```python
from build123d import *

# Parameters (mm, degrees)
F1_DEPTH        = 17.5
F2_DEPTH        = 12
F3_DEPTH        = 3.5
F4_R            = 10
F7_R            = 10
F11_D           = 9
F13_D           = 9
F20_D           = 5.5
F20_DEPTH       = 3.5
F20_CSINK_D     = 8
F20_CSINK_ANGLE = 82
F20_TIP         = 1.6523667023
F22_D           = 5.5
F22_DEPTH       = 3.5
F22_CSINK_D     = 8
F22_CSINK_ANGLE = 82
F22_TIP         = 1.6523667023
F24_DEPTH       = 2.5


with BuildPart() as f1:
    # F0 (on Front) → F1 (new body, symmetric)
    with BuildSketch(Plane.XZ):
        Polygon((52, -6), (52, 6), (23.1059112473, 6), (16.606986017, 6), (9.0432994782, 6), (7.106986017, 6), (-9.5, 6), (-29.3893709637, 6), (-52, 6), (-52, -6), align=None)
    extrude(amount=F1_DEPTH, both=True)

    # F0 (on Front) → F2 (join, symmetric)
    with BuildSketch(Plane.XZ):
        with BuildLine():
            ThreePointArc((-24.5597418322, 9.7059047745), (-26.3455638186, 7.0332332985), (-29.3893709637, 6))
            Line((-29.3893709637, 6), (-9.5, 6))
            Line((-9.5, 6), (-9.5, 26))
            Line((-9.5, 26), (-15, 26))
            ThreePointArc((-15, 26), (-17.9660849945, 25.5499916129), (-20.665217364, 24.2404679611))
            Line((-20.665217364, 24.2404679611), (-24.5597418322, 9.7059047745))
        make_face()
        with BuildLine():
            ThreePointArc((-11, 16), (-17.8284271247, 13.1715728753), (-15, 20))
            ThreePointArc((-15, 20), (-12.1715728753, 18.8284271247), (-11, 16))
        make_face(mode=Mode.SUBTRACT)
        with BuildLine():
            Line((-9.5, 6), (7.106986017, 6))
            ThreePointArc((7.106986017, 6), (4.7982429508, 6.5649458341), (3.0112257955, 8.1321178182))
            Line((3.0112257955, 8.1321178182), (-9.5, 26))
            Line((-9.5, 26), (-9.5, 6))
        make_face()
        with BuildLine():
            Line((9.0432994782, 6), (16.606986017, 6))
            ThreePointArc((16.606986017, 6), (14.2982429508, 6.5649458341), (12.5112257955, 8.1321178182))
            Line((12.5112257955, 8.1321178182), (0, 26))
            Line((0, 26), (-9.5, 26))
            Line((-9.5, 26), (3.0112257955, 8.1321178182))
            ThreePointArc((3.0112257955, 8.1321178182), (4.7982429508, 6.5649458341), (7.106986017, 6))
            Line((7.106986017, 6), (9.0432994782, 6))
        make_face()
    extrude(amount=F2_DEPTH, both=True)

    # F0 (on Front) → F3 (join, symmetric)
    with BuildSketch(Plane.XZ):
        with BuildLine():
            Line((16.606986017, 6), (23.1059112473, 6))
            ThreePointArc((23.1059112473, 6), (20.7971681811, 6.5649458341), (19.0101510258, 8.1321178182))
            Line((19.0101510258, 8.1321178182), (-2.4481396714, 38.7777329056))
            ThreePointArc((-2.4481396714, 38.7777329056), (-10.4179907667, 42.9471562808), (-17.2274066103, 37.0705523608))
            Line((-17.2274066103, 37.0705523608), (-20.665217364, 24.2404679611))
            ThreePointArc((-20.665217364, 24.2404679611), (-17.9660849945, 25.5499916129), (-15, 26))
            Line((-15, 26), (-9.5, 26))
            Line((-9.5, 26), (0, 26))
            Line((0, 26), (12.5112257955, 8.1321178182))
            ThreePointArc((12.5112257955, 8.1321178182), (14.2982429508, 6.5649458341), (16.606986017, 6))
        make_face()
        with BuildLine():
            ThreePointArc((-6.75, 35), (-7.5554563517, 33.0554563517), (-9.5, 32.25))
            ThreePointArc((-9.5, 32.25), (-11.4445436483, 36.9445436483), (-6.75, 35))
        make_face(mode=Mode.SUBTRACT)
    extrude(amount=F3_DEPTH, both=True)

    # F8: sweep along a path in F5
    with BuildLine(Plane.XZ.offset(12)) as f8_path:
        Line((0, 26), (14.0041507642, 6))
    # F4 (on face) → F8 (sweep, cut)
    with BuildSketch(Plane.XY.offset(26)):
        with Locations((0, -13.5)):
            Circle(F4_R)
    sweep(path=f8_path.line, mode=Mode.SUBTRACT)

    # F9: sweep along a path in F6
    with BuildLine(Plane(origin=(0, 12, 0), x_dir=(-1, 0, 0), z_dir=(0, 1, 0))) as f9_path:
        Line((0, 26), (-14.0041507642, 6))
    # F7 (on face) → F9 (sweep, cut)
    with BuildSketch(Plane.XY.offset(26)):
        with Locations((0, 13.5)):
            Circle(F7_R)
    sweep(path=f9_path.line, mode=Mode.SUBTRACT)

    # F11 (through all)
    with Locations(Plane.XY.offset(6)):
        with Locations((40, 0)):
            Hole(F11_D / 2)

    # F13 (through all)
    with Locations(Plane.XY.offset(6)):
        with Locations((-40, 0)):
            Hole(F13_D / 2)

    # F15: sweep along a path in F15_path
    with BuildLine(Plane(origin=(-52, -17.5, -6), x_dir=(0, 0, -1), z_dir=(0, 1, 0))) as f15_path:
        Line((0, 0), (-12, 0))
    # F14 (on face) → F15 (sweep, cut)
    with BuildSketch(Plane.XY.offset(6)):
        with BuildLine():
            Line((-45.3612986682, 10.6920782903), (-32, 17.5))
            Line((-32, 17.5), (-52, 17.5))
            Line((-52, 17.5), (-52, -17.5))
            Line((-52, -17.5), (-32, -17.5))
            Line((-32, -17.5), (-45.3612986682, -10.6920782903))
            ThreePointArc((-45.3612986682, -10.6920782903), (-51.9134126713, 0), (-45.3612986682, 10.6920782903))
        make_face()
    sweep(path=f15_path.line, mode=Mode.SUBTRACT)

    # F16: sweep along a path in F0
    with BuildLine(Plane.XZ) as f16_path:
        Line((-52, 6), (-52, -6))
    # F12 (on face) → F16 (sweep, cut)
    with BuildSketch(Plane.XY.offset(6)):
        with BuildLine():
            ThreePointArc((-40, -4.5), (-44.5, 0), (-40, 4.5))
            Line((-40, 4.5), (-52, 4.5))
            Line((-52, 4.5), (-52, -4.5))
            Line((-52, -4.5), (-40, -4.5))
        make_face()
    sweep(path=f16_path.line, mode=Mode.SUBTRACT)

    # F17: sweep along a path in F17_path
    with BuildLine(Plane(origin=(52, 17.5, 6), x_dir=(0, 0, 1), z_dir=(0, -1, 0))) as f17_path:
        Line((0, 0), (-12, 0))
    # F12 (on face) → F17 (sweep, cut)
    with BuildSketch(Plane.XY.offset(6)):
        with BuildLine():
            Line((45.3612986682, -10.6920782903), (32, -17.5))
            Line((32, -17.5), (52, -17.5))
            Line((52, -17.5), (52, -4.4991668823))
            Line((52, -4.4991668823), (51.0380473784, -4.4991668823))
            ThreePointArc((51.0380473784, -4.4991668823), (48.7593240742, -8.1086282103), (45.3612986682, -10.6920782903))
        make_face()
    sweep(path=f17_path.line, mode=Mode.SUBTRACT)

    # F18: sweep along a path in F18_path
    with BuildLine(Plane(origin=(52, 17.5, 6), x_dir=(0, 0, 1), z_dir=(0, -1, 0))) as f18_path:
        Line((0, 0), (-12, 0))
    # F12 (on face) → F18 (sweep, cut)
    with BuildSketch(Plane.XY.offset(6)):
        with BuildLine():
            ThreePointArc((51.0380473784, -4.4991668823), (51.9134126713, 0), (51.0380473784, 4.4991668823))
            Line((51.0380473784, 4.4991668823), (40.0865873287, 4.4991668823))
            ThreePointArc((40.0865873287, 4.4991668823), (43.2124478968, 3.1512185755), (44.5, 0))
            ThreePointArc((44.5, 0), (43.2124478968, -3.1512185755), (40.0865873287, -4.4991668823))
            Line((40.0865873287, -4.4991668823), (51.0380473784, -4.4991668823))
        make_face()
        with BuildLine():
            Line((52, 4.4991668823), (51.0380473784, 4.4991668823))
            ThreePointArc((51.0380473784, 4.4991668823), (51.9134126713, 0), (51.0380473784, -4.4991668823))
            Line((51.0380473784, -4.4991668823), (52, -4.4991668823))
            Line((52, -4.4991668823), (52, 4.4991668823))
        make_face()
        with BuildLine():
            Line((52, 17.5), (32, 17.5))
            Line((32, 17.5), (45.3612986682, 10.6920782903))
            ThreePointArc((45.3612986682, 10.6920782903), (48.7593240742, 8.1086282103), (51.0380473784, 4.4991668823))
            Line((51.0380473784, 4.4991668823), (52, 4.4991668823))
            Line((52, 4.4991668823), (52, 17.5))
        make_face()
    sweep(path=f18_path.line, mode=Mode.SUBTRACT)

    # F20
    with Locations(Plane.XZ.offset(3.5)):
        with Locations((-9.5, 35)):
            CounterSinkHole(F20_D / 2, F20_CSINK_D / 2, depth=F20_DEPTH, counter_sink_angle=F20_CSINK_ANGLE)
            with Locations((0, 0, -(F20_DEPTH + F20_TIP / 2))):  # 118° drill point
                Cone(0, F20_D / 2, F20_TIP, mode=Mode.SUBTRACT)

    # F22
    with Locations(Plane(origin=(0, 3.5, 0), x_dir=(-1, 0, 0), z_dir=(0, 1, 0))):
        with Locations((9.5, 35)):
            CounterSinkHole(F22_D / 2, F22_CSINK_D / 2, depth=F22_DEPTH, counter_sink_angle=F22_CSINK_ANGLE)
            with Locations((0, 0, -(F22_DEPTH + F22_TIP / 2))):  # 118° drill point
                Cone(0, F22_D / 2, F22_TIP, mode=Mode.SUBTRACT)

    # F23 (on Front) → F24 (cut, symmetric)
    with BuildSketch(Plane.XZ):
        Polygon((-13.4935649536, 32.709419195), (-9.5146586694, 30.3951730687), (-5.5210095913, 32.6838839269), (-5.5062667973, 37.2868409115), (-9.4851730816, 39.6010870379), (-13.4788221597, 37.3123761796), align=None)
    extrude(amount=F24_DEPTH, both=True, mode=Mode.SUBTRACT)


solid = f1.part
```
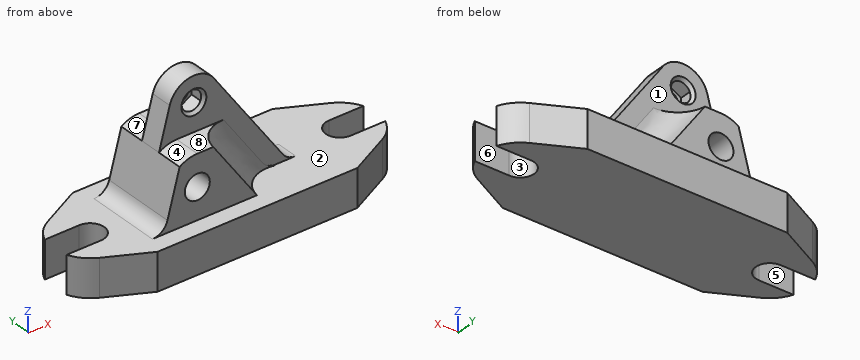
Check sheet for the modelled part. Datum: model origin and axes. Units: mm. Face numbers are marked on the shaded views. A direction names the side the tool comes from. Give positions to 0.01 mm unless a question says otherwise; leave off trailing zeros. Write each loop counter-clockwise with the first axis right and the second up, starting at its lowest first coordinate (ties: lowest second). Pieces come first, ordered by that corner, then holes.
Item 1: Cross-section at B-B (x = -42). Enter the section's corners in (y, z), and give its area (3 significant figures).
Item 2: Access from +Z, -Z, +X, -X, +Y, -Y to the whole of each face (thin tool, end or side, straight path). Record for the marked faces 4, 5, 6, 7 and 8.
Item 3: Cross-section at D-D (x = 20.5). Enter the section's corners in (y, z).
Item 4: Gauge pin test, flat ends, axial feed: pin 1 (5.5 mm diameter, centred on x = 48.5, z = -1, fed in from -Y); pin 2 (4 mm diameter, centred on x = -8.5, z = 33.5, fed in from +Y); pin 3 (3 mm diameter, centred on y = 8, z = 3.5, fed in from -X); pin 4 (16 mm diameter, centred on x = -18.5, z = 12, fed in from +Y). Record the tip position at first contact, or that the pin passes through.
Item 5: Scan lines: L1, parallel to Z at x = -15, y = -4; L2, parallel to Y at x = 7, z = 16; L3, parallel to Z at x = -46.5, y = -6. Record each from-to range of solid material in increasing order.
Item 6: Cross-section at A-A (y = 1.5). Enter the section's corners in (x, z).
Item 7: Draft check along Y on the marked faces 1, 2 and 3. Enter one of: released by +Y, released by -Y, zero draft, split by the parting line, or undercut.
Item 8: Cross-section at C-C (z = 4.5). Enter the section's corners in (x, y), and give its area (3 significant figures).
Report:
1. outline: (-12.4, -6) - (-4.5, -6) - (-4.5, 6) - (-12.4, 6) - close; (4.5, -6) - (12.4, -6) - (12.4, 6) - (4.5, 6) - close
1. area: 190 mm2
2. face 4: +Z, -X, -Y
2. face 5: +Z, -Z, -X
2. face 6: +Z, -Z, +X
2. face 7: +Z, -X, +Y
2. face 8: +Z, +X, -X, -Y
3. outline: (-17.5, -6) - (17.5, -6) - (17.5, 6) - (3.5, 6) - (3.5, 6.73) - (-3.5, 6.73) - (-3.5, 6) - (-17.5, 6) - close
4. pin 1: stops at y = -10.48
4. pin 2: stops at y = 3.27
4. pin 3: stops at x = -50
4. pin 4: stops at y = 17.5
5. L1: z = -6 to 12, 20 to 26
5. L2: y = -3.5 to 3.5
5. L3: z = -6 to 6
6. outline: (-35.76, -6) - (35.76, -6) - (35.76, 6) - (23.11, 6) arc R5 cw to (19.01, 8.13) - (-2.45, 38.78) arc R8 ccw to (-17.23, 37.07) - (-24.56, 9.71) arc R5 cw to (-29.39, 6) - (-35.76, 6) - close; hole circle Ø8 at (-15, 16); hole (-13.49, 32.71) - (-9.51, 30.4) - (-5.52, 32.68) - (-5.51, 37.29) - (-9.49, 39.6) - (-13.48, 37.31) - close
7. face 1: released by +Y
7. face 2: zero draft
7. face 3: undercut
8. outline: (-51.04, -4.5) arc R12 ccw to (-45.36, -10.69) - (-32, -17.5) - (32, -17.5) - (45.36, -10.69) arc R12 ccw to (51.04, -4.5) - (40.09, -4.5) arc R4.5 cw (long way) to (40.09, 4.5) - (51.04, 4.5) arc R12 ccw to (45.36, 10.69) - (32, 17.5) - (-32, 17.5) - (-45.36, 10.69) arc R12 ccw to (-51.04, 4.5) - (-40, 4.5) arc R4.5 cw to (-40, -4.5) - close
8. area: 2,920 mm2
